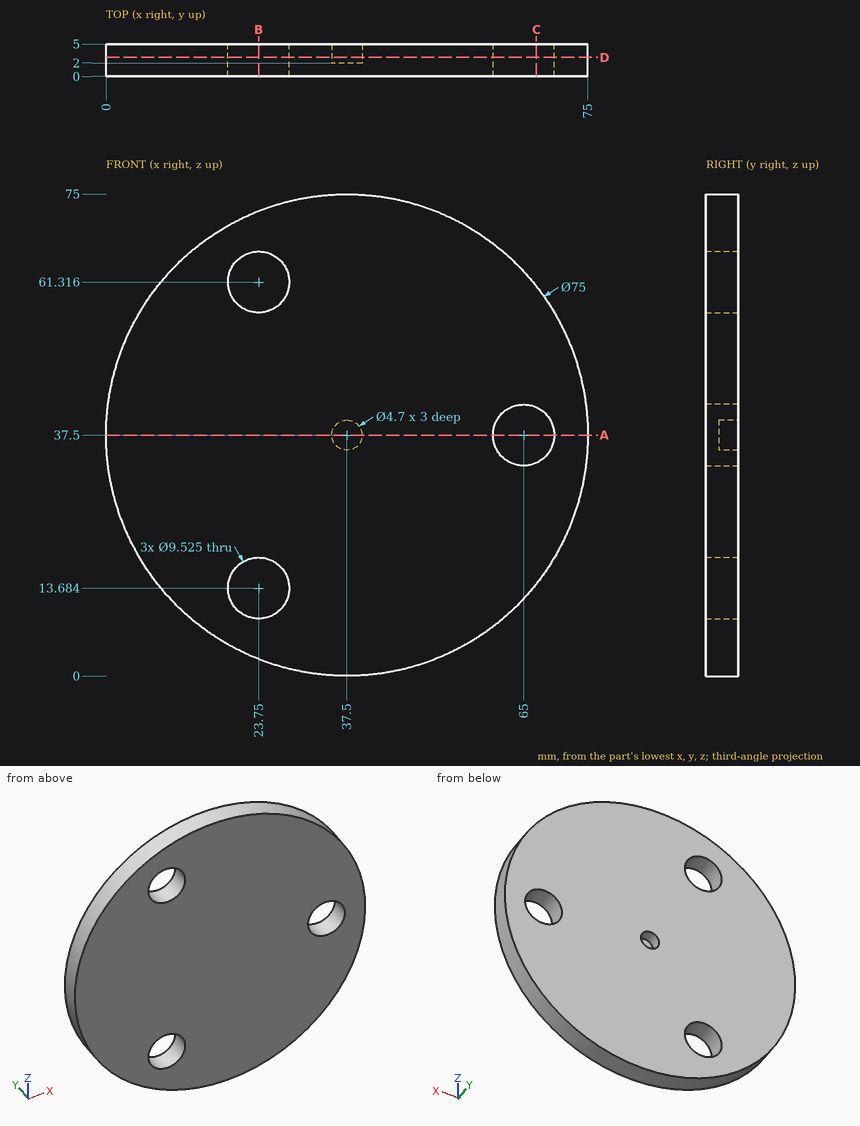
Study the drawing (mm; zero at the part's minimum x, y, z) and answer. Round coordinates to 2 decimals unless told otherwise and drop trailing zeros. Loops run counter-clockwise (first coordinate to the right, second up) from the corner with the lowest first, then second, coordinate; pieces in that order, holes last.
Q1. Section D-D, the plane y = 2.9 is taken. Count the separate pieces of the cut face and the enclosed holes in it, then the cut area to 3 significant figures.
Q2. Section A-A, the plane z = 37.5 is taken. Determine the outline of the cut face in (x, y), then the cut area to 3 significant figures.
Q3. Section C-C, the plane x = 67 is taken. Determine the outline of the cut face in (y, z), then the cut area to 3 significant figures.
Q4. Find the intervals of material crossed by line 1 (X direction, y = 3.6, z = 39.5) (1 decimal); line 2 (X direction, y = 1.75, z = 37.5); line 3 (X direction, y = 0.7, z = 10) (1 decimal), in increasing order.
Q5. Section B-B, the plane x = 23.75 is taken. Determine the outline of the cut face in (y, z).
Q6. Given pin 1 Ø2 at (x, z) = (58.5, 46) entering from -Y; pin 2 Ø2 at (y, z) = (3, 67.5) entering from -X (1 decimal); pin 3 Ø2 at (x, y) = (47, 2) entering from -Z; pin 4 Ø2 at (x, y) = (21, 2) entering from +Z, each flat-ended and moving along its own axis, determine where each tip first touches the part or whether it passes through.
Completed:
1. separate pieces: 1
1. enclosed holes: 4
1. area: 4,190 mm2
2. outline: (0, 0) - (60.24, 0) - (60.24, 5) - (39.85, 5) - (39.85, 2) - (35.15, 2) - (35.15, 5) - (0, 5) - close; (69.76, 0) - (75, 0) - (75, 5) - (69.76, 5) - close
2. area: 313 mm2
3. outline: (0, 14.35) - (5, 14.35) - (5, 33.18) - (0, 33.18) - close; (0, 41.82) - (5, 41.82) - (5, 60.65) - (0, 60.65) - close
3. area: 188 mm2
4. line 1: x = 0.1 to 36.3, 38.7 to 60.7, 69.3 to 74.9
4. line 2: x = 0 to 60.24, 69.76 to 75
4. line 3: x = 12 to 20.7, 26.8 to 63
5. outline: (0, 2.61) - (5, 2.61) - (5, 8.92) - (0, 8.92) - close; (0, 18.45) - (5, 18.45) - (5, 56.55) - (0, 56.55) - close; (0, 66.08) - (5, 66.08) - (5, 72.39) - (0, 72.39) - close
6. pin 1: stops at y = 0
6. pin 2: stops at x = 13.7
6. pin 3: stops at z = 0.98
6. pin 4: stops at z = 71.65
